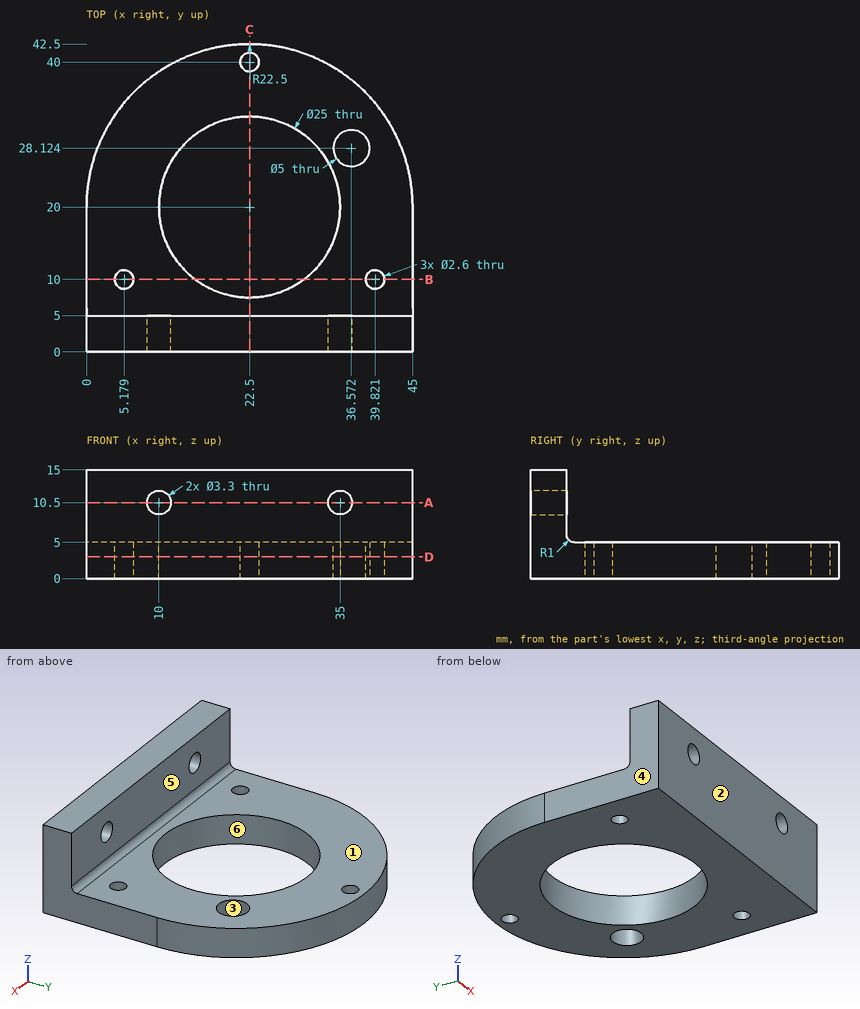
The drawing under review shows one solid part. Ordinate dimensions are in mm from its lowest x, y, z. A direction names the side the tool comes from. Coordinates: 2 decimals unless noted, no trailing zeros. Write each loop counter-clockwise with the first axis right and the second up, starting at its lowest first coordinate (ties: lowest second). Pieces come first, ordered by that corner, then holes. Notation, with made-up numbers: (10, 14.25) - (55, 14.25) arc R19 cw to (55, 23.25) - close; hole circle Ø9 at (70.25, 23). An arc over 180 degrees is marked (long way). Answer in a Markdown table with one row per item. Add a question column.
Q1. We need section A-A, the plane z = 10.5. State the section outline as (x, y) points.
Q2. We need section D-D, the plane z = 3. State the section outline as (x, y) points (1 decimal).
Q3. We need section C-C, the plane x = 22.5. State the section outline as (y, z) points.
Q4. We need section B-B, the plane y = 10. State the section outline as (x, z) points, and give its area (3 significant figures).
Q5. Draft analysis for pull direction Y (two halves, no side actions). For the marked faces 3, 4, 5 and 6, state which applies: +Y half, -Y half, draft (parallel to the pull), parting line (faces both ways), or undercut.
Q6. For probe 1 along Y at (x, z) = (22.5, 2.2); probe 2 along X at (y, z) = (20, 3.4); probe 3 along X at (y, z) = (10.5, 3.5) (1 decimal), list the stretches that pass through material, from the lowest coordinate up.
Q7. Tool access review of the marked faces 1 and 2: name each direction out of +Z, -Z, +X, -X, +Y, -Y from which nothing blocks a thin tool from reaching the whole face with its end or side.
Q8. For P1, Ø10, axis at x = 23.5, y = 15, coming from the -Z side; P2, Ø4, axis at x = 39.5, y = 33.5, coming from the -Z side; P3, Ø1, axis at x = 25, z = 4, coming from the +Y side; P4, Ø3, axis at x = 39.82, y = 10, coming from the +Z side, all flat-tipped, find the tip position at first contact; note any pin that passes through.
Answer list:
| question | item | result |
|---|---|---|
| 1 | outline | (0, 0) - (8.35, 0) - (8.35, 5) - (0, 5) - close; (11.65, 0) - (33.35, 0) - (33.35, 5) - (11.65, 5) - close; (36.65, 0) - (45, 0) - (45, 5) - (36.65, 5) - close |
| 2 | outline | (0, 0) - (45, 0) - (45, 20) arc R22.5 ccw to (0, 20) - close; hole circle Ø2.6 at (5.2, 10); hole circle Ø25 at (22.5, 20); hole circle Ø2.6 at (22.5, 40); hole circle Ø5 at (36.6, 28.1); hole circle Ø2.6 at (39.8, 10) |
| 3 | outline | (0, 0) - (7.5, 0) - (7.5, 5) - (6, 5) arc R1 cw to (5, 6) - (5, 15) - (0, 15) - close; (32.5, 0) - (38.7, 0) - (38.7, 5) - (32.5, 5) - close; (41.3, 0) - (42.5, 0) - (42.5, 5) - (41.3, 5) - close |
| 4 | outline | (0, 0) - (3.88, 0) - (3.88, 5) - (0, 5) - close; (6.48, 0) - (15, 0) - (15, 5) - (6.48, 5) - close; (30, 0) - (38.52, 0) - (38.52, 5) - (30, 5) - close; (41.12, 0) - (45, 0) - (45, 5) - (41.12, 5) - close |
| 4 | area | 124 mm2 |
| 5 | face 3 | undercut |
| 5 | face 4 | draft |
| 5 | face 5 | +Y half |
| 5 | face 6 | undercut |
| 6 | probe 1 | y = 0 to 7.5, 32.5 to 38.7, 41.3 to 42.5 |
| 6 | probe 2 | x = 0 to 10, 35 to 45 |
| 6 | probe 3 | x = 0 to 4, 6.4 to 14.4, 30.6 to 38.6, 41 to 45 |
| 7 | face 1 | +Z, +X, -X, +Y |
| 7 | face 2 | +Z, -Z, +X, -X, -Y |
| 8 | P1 | passes through |
| 8 | P2 | stops at z = 0 |
| 8 | P3 | stops at y = 42.41 |
| 8 | P4 | stops at z = 5 |
